from build123d import *

# Parameters (mm, degrees)
SKETCH1_W           = 123
SKETCH1_H           = 56
SKETCH1_W_2         = 115
SKETCH1_H_2         = 48
BOSS_EXTRUDE1_DEPTH = 4
SKETCH1_3_W         = 123
SKETCH1_3_H         = 56
SKETCH1_3_W_2       = 115
SKETCH1_3_H_2       = 48
BOSS_EXTRUDE2_DEPTH = 49
SKETCH2_W           = 123
SKETCH2_H           = 5
BOSS_EXTRUDE3_DEPTH = 15
BOSS_EXTRUDE4_DEPTH = 5
CUT_EXTRUDE1_DEPTH  = 136.329228181
CUT_EXTRUDE2_DEPTH  = 136.329228181
CUT_EXTRUDE3_DEPTH  = 5
FILLET5_R           = 3.5
FILLET6_R           = 3.5
FILLET7_R           = 3.5
FILLET8_R           = 3.5
SKETCH8_R           = 1.75
CUT_EXTRUDE4_DEPTH  = 89.565300892


with BuildPart() as part:
    # Sketch1 → Boss-Extrude1 (new body)
    with BuildSketch(Plane.XY):
        Rectangle(SKETCH1_W, SKETCH1_H)
        Rectangle(SKETCH1_W_2, SKETCH1_H_2, mode=Mode.SUBTRACT)
        Rectangle(SKETCH1_W_2, SKETCH1_H_2)
    extrude(amount=BOSS_EXTRUDE1_DEPTH)

    # Sketch1_3 → Boss-Extrude2 (add)
    with BuildSketch(Plane.XY):
        Rectangle(SKETCH1_3_W, SKETCH1_3_H)
        Rectangle(SKETCH1_3_W_2, SKETCH1_3_H_2, mode=Mode.SUBTRACT)
    extrude(amount=BOSS_EXTRUDE2_DEPTH)

    # Sketch2 → Boss-Extrude3 (add)
    with BuildSketch(Plane(origin=(0, 0, 0), x_dir=(-1, 0, 0), z_dir=(0, 0, -1))):
        with Locations((0, -10.25)):
            Rectangle(SKETCH2_W, SKETCH2_H)
        with Locations((0, 10.25)):
            Rectangle(SKETCH2_W, SKETCH2_H)
    extrude(amount=BOSS_EXTRUDE3_DEPTH)

    # Sketch3 → Boss-Extrude4 (add)
    with BuildSketch(Plane(origin=(61.5, 0, 0), x_dir=(0, 0, -1), z_dir=(1, 0, 0))):
        Polygon((0, -28), (15, -12.75), (0, -12.75), align=None)
        Polygon((15, 12.75), (0, 28), (0, 12.75), align=None)
    boss_extrude4 = extrude(amount=-BOSS_EXTRUDE4_DEPTH)

    # Mirror1: Boss-Extrude4 across plane
    add(boss_extrude4.mirror(Plane.ZY))

    # Sketch4 → Cut-Extrude1 (cut, through all)
    with BuildSketch(Plane.ZY.offset(61.5)):
        Polygon((19, 28), (49, -24), (49, 24), (49, 28), align=None)
    extrude(amount=-CUT_EXTRUDE1_DEPTH, mode=Mode.SUBTRACT)

    # Sketch6 → Cut-Extrude2 (cut, through all)
    with BuildSketch(Plane.ZY.offset(61.5)):
        Polygon((12.66631443, -19), (30.66362763, -2.222508572), (40.342949608, -19), align=None)
        Polygon((28.088718183, 2.240667802), (18.419872685, 19), (9, 19), (9, -15.582181004), (27.67670193, 1.828651549), align=None)
    extrude(amount=-CUT_EXTRUDE2_DEPTH, mode=Mode.SUBTRACT)

    # Sketch7 → Cut-Extrude3 (cut)
    with BuildSketch(Plane.XZ.offset(28)):
        Polygon((0, 16.698332058), (28.496575704, 39), (-28.496575704, 39), align=None)
        Polygon((-47.5, 28.475580986), (-29.003424296, 14), (-12.777777778, 14), (-47.5, 41.173913043), align=None)
        Polygon((12.777777778, 14), (29.003424296, 14), (47.5, 28.475580986), (47.5, 41.173913043), align=None)
    extrude(amount=-CUT_EXTRUDE3_DEPTH, mode=Mode.SUBTRACT)

    # Fillet5
    fillet5_edges = [part.edges().sort_by_distance(p)[0] for p in [
        (29.003424296, -26, 14),
        (12.777777778, -26, 14),
        (47.5, -26, 41.173913043),
        (47.5, -26, 28.475580986),
        (-29.003424296, -26, 14),
        (-47.5, -26, 28.475580986),
        (-47.5, -26, 41.173913043),
        (-12.777777778, -26, 14),
        (28.496575704, -26, 39),
        (0, -26, 16.698332058),
        (-28.496575704, -26, 39),
    ]]
    fillet(fillet5_edges, radius=FILLET5_R)

    # Fillet6
    fillet6_edges = [part.edges().sort_by_distance(p)[0] for p in [
        (-59.5, 19, 18.419872685),
        (-59.5, 19, 9),
        (-59.5, -15.582181004, 9),
        (-59.5, -19, 12.66631443),
        (-59.5, -19, 40.342949608),
        (-59.5, -2.222508572, 30.66362763),
        (-59.5, 2.240667802, 28.088718183),
        (59.5, -2.222508572, 30.66362763),
        (59.5, 2.240667802, 28.088718183),
        (59.5, -19, 40.342949608),
        (59.5, 19, 9),
        (59.5, 19, 18.419872685),
        (59.5, -19, 12.66631443),
        (59.5, -15.582181004, 9),
    ]]
    fillet(fillet6_edges, radius=FILLET6_R)

    # Fillet7
    fillet7_edges = [part.edges().sort_by_distance(p)[0] for p in [
        (-57.5, 24, 12.653846154),
        (57.5, 24, 12.653846154),
        (-57.5, -24, 26.5),
        (57.5, -24, 26.5),
    ]]
    fillet(fillet7_edges, radius=FILLET7_R)

    # Fillet8
    fillet8_edges = [part.edges().sort_by_distance(p)[0] for p in [
        (-61.5, 28, 9.5),
        (61.5, 28, 9.5),
        (61.5, -28, 24.5),
        (-61.5, -28, 24.5),
    ]]
    fillet(fillet8_edges, radius=FILLET8_R)

    # Sketch8 → Cut-Extrude4 (cut, through all)
    with BuildSketch(Plane(origin=(0, 12.75, 0), x_dir=(1, 0, 0), z_dir=(0, 1, 0))):
        with Locations(Location((40, 7.5, 0), (0, 0, 270))):
            Circle(SKETCH8_R)
        with Locations(Location((-40, 7.5, 0), (0, 0, 90))):
            Circle(SKETCH8_R)
    extrude(amount=-CUT_EXTRUDE4_DEPTH, mode=Mode.SUBTRACT)


solid = part.part
The listing builds one solid part. Answer for the finished solid, in the listing's coordinates (mm). A direction names the side the tool comes from. Coordinates: 2 decimals unless noted, no trailing zeros. Order: outer loops, then holes, each group sorted by start corner. A loop starts at its lowest first (then second) coordinate and runs counter-clockwise, first axis right, second up. Notation, with made-up numbers: (43.5, -30) -> (93.5, -30) arc R21 ccw to (93.5, -9) -> close; hole circle Ø5 at (36.5, -14.5). An arc over 180 degrees is marked (long way). Answer in a Markdown table with one row per item. Add a question column.
Item 1: Each of these flat-tipped pins is pushed along its axis until it touches: P1, Ø6, axis at x = 33.5, y = 2.5, coming from the +Z side; P2, Ø2, axis at y = -11.5, z = 34, coming from the -X side; P3, Ø4.5, axis at y = -20.5, z = -10, coming from the -X side; P4, Ø4.5, axis at x = 27, z = -11, coming from the -Y side. Where does it stop, or does it pass through?
Item 2: Find the intervals of material crossed by L1, parallel to X at y = -8.9, z = -7.5; L2, parallel to Y at x = 43.5, z = 10.5; L3, parallel to Z at x = -40, y = -11, in increasing order. Write a range as from..to.
Item 3: Find section C-C (y = -3). Write down the section's boundary in (x, z), then the cut area to 3 significant figures.
Item 4: Find section B-B (x = -40). Write down the section's boundary in (y, z), then the cut area to 3 significant figures.
Item 5: Find section A-A (z = 6). Write down the section's boundary in (x, y).
Item 6: Which of the six approach directions +Z, -Z, +X, -X, +Y, -Y give full straight-line access (tool end or side, diameter ignored) to faces 4 (the face through (59.53, -4.33, 30.39)), 5 (the face through (-1, 24, 13)), 6 (the face through (47.5, -26, 32))?
Item 7: Determine the mould class of faces 1 (the face through (61.5, -11, 10)), 2 (the face through (56.5, 17, -4)), 3 (the face through (-59.472, -16.728, 18.276)) for opening direction X: +X half, -X half, draft (parallel to the pull), parting line (faces both ways), or undercut.
Item 8: Find section D-D (z = -7.5). State how many separate pieces and enclosed holes the cut face has, then the cut area to 3 significant figures.
Result set:
| question | item | result |
|---|---|---|
| 1 | P1 | stops at z = 4 |
| 1 | P2 | passes through |
| 1 | P3 | stops at x = -61.5 |
| 1 | P4 | stops at y = -12.75 |
| 2 | L1 | x = -61.5..-41.75, -38.25..38.25, 41.75..61.5 |
| 2 | L2 | y = -28..-24, 24..28 |
| 2 | L3 | z = -15..-9.25, -5.75..4 |
| 3 | outline | (-61.5, 0) -> (61.5, 0) -> (61.5, 9) -> (57.5, 9) -> (57.5, 4) -> (-57.5, 4) -> (-57.5, 9) -> (-61.5, 9) -> close; (-61.5, 22.5) -> (-57.5, 22.5) -> (-57.5, 36.88) -> (-61.5, 36.88) -> close; (57.5, 22.5) -> (61.5, 22.5) -> (61.5, 36.88) -> (57.5, 36.88) -> close |
| 3 | area | 647 mm² |
| 4 | outline | (-28, 0) -> (-12.75, 0) -> (-12.75, -5.75) -> (-7.75, -5.75) -> (-7.75, 0) -> (7.75, 0) -> (7.75, -5.75) -> (12.75, -5.75) -> (12.75, 0) -> (28, 0) -> (28, 19) -> (24, 21.31) -> (24, 4) -> (-24, 4) -> (-24, 22.61) -> (-28, 22.61) -> close; (-28, 35.3) -> (-24, 35.3) -> (-24, 49) -> (-28, 49) -> close; (-12.75, -15) -> (-7.75, -15) -> (-7.75, -9.25) -> (-12.75, -9.25) -> close; (7.75, -15) -> (12.75, -15) -> (12.75, -9.25) -> (7.75, -9.25) -> close |
| 4 | area | 533 mm² |
| 5 | outline | (-61.5, -24.5) arc R3.5 ccw to (-58, -28) -> (58, -28) arc R3.5 ccw to (61.5, -24.5) -> (61.5, 24.5) arc R3.5 ccw to (58, 28) -> (-58, 28) arc R3.5 ccw to (-61.5, 24.5) -> close; hole (-57.5, -20.5) arc R3.5 ccw to (-54, -24) -> (54, -24) arc R3.5 ccw to (57.5, -20.5) -> (57.5, 20.5) arc R3.5 ccw to (54, 24) -> (-54, 24) arc R3.5 ccw to (-57.5, 20.5) -> close |
| 6 | face 4 | +X, -X |
| 6 | face 5 | +Z |
| 6 | face 6 | +Y, -Y |
| 7 | face 1 | +X half |
| 7 | face 2 | undercut |
| 7 | face 3 | draft |
| 8 | separate pieces | 6 |
| 8 | enclosed holes | 0 |
| 8 | area | 1,310 mm² |
